Source: three-view drawing plus pictorial views. Frame: mm from the lowest corner of the part. A direction names the side the tool comes from. Round coordinates to 2 decimals unless told otherwise and drop trailing zeros. Loops run counter-clockwise (first coordinate to the right, second up) from the corner with the lowest first, then second, coordinate; pieces in that order, holes last. Notation, with made-up numbers: M 76,53 L 87,53 A17 cw 87,66 Z; hole C 60,-25 d11. An arc over 180 degrees is marked long. Write each question's results on one line, items separated by ' | '.
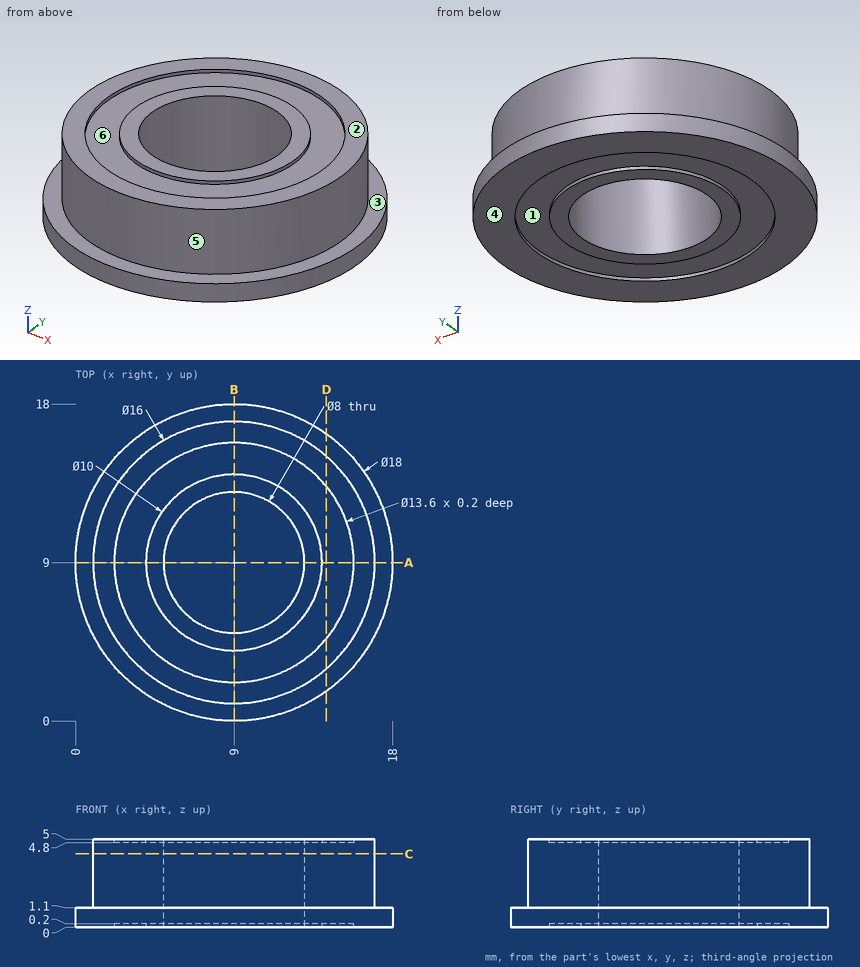
1. Access query for the marked faces 1, 2 and 3. Directions: +Z, -Z, +X, -X, +Y, -Y. A direction counts if a zero-diameter tool reaches every point of the face in a straight line with its end or side. Return the directions, or none.
Answer key:
face 1: -Z | face 2: +Z, +X, -X, +Y, -Y | face 3: +Z
2. Section D-D (x = 14.25). Output: boundary loops of the cut face in (y, z), then the cut area to 3 significant figures.
Answer key:
outline: M 1.69,0 L 4.68,0 L 4.68,0.2 L 13.32,0.2 L 13.32,0 L 16.31,0 L 16.31,1.1 L 15.04,1.1 L 15.04,5 L 13.32,5 L 13.32,4.8 L 4.68,4.8 L 4.68,5 L 2.96,5 L 2.96,1.1 L 1.69,1.1 Z | area: 59.7 mm²
3. Section C-C (z = 4.15). Output: boundary loops of the cut face in (x, y), then the cut area to 3 significant figures.
Answer key:
outline: C 9,9 d16; hole C 9,9 d8 | area: 151 mm²
4. Ray query, probe 1 along Y at (x, z) = (9, 0.15); probe 2 along Y at (x, z) = (9, 2.8); probe 3 along Y at (x, z) = (11.25, 2.2). Return the intervals inside material, ascending.
Answer key:
probe 1: y = 0 to 2.2, 4 to 5, 13 to 14, 15.8 to 18 | probe 2: y = 1 to 5, 13 to 17 | probe 3: y = 1.32 to 5.69, 12.31 to 16.68
5. Section A-A (y = 9). Output: boundary loops of the cut face in (x, z).
Answer key:
outline: M 0,0 L 2.2,0 L 2.2,0.2 L 4,0.2 L 4,0 L 5,0 L 5,5 L 4,5 L 4,4.8 L 2.2,4.8 L 2.2,5 L 1,5 L 1,1.1 L 0,1.1 Z; M 13,0 L 14,0 L 14,0.2 L 15.8,0.2 L 15.8,0 L 18,0 L 18,1.1 L 17,1.1 L 17,5 L 15.8,5 L 15.8,4.8 L 14,4.8 L 14,5 L 13,5 Z
6. Pin query (flat end, axial travel): P1, Ø9, axis at x = 5.5, y = 9, coming from the +Z side; P2, Ø6.5, axis at x = 9, y = 9, coming from the -Z side; P3, Ø1, axis at y = 2, z = 4.5, coming from the -X side. Return the tip coordinate at first contact, or that it passes through.
Answer key:
P1: stops at z = 5 | P2: passes through | P3: stops at x = 4.34
7. Draft query along Y for the marked faces 4, 5 and 6. Return one class per face: pulls with the +Y half, pulls with the -Y half, needs draft (parallel to the pull), parting line crosses it, or undercut.
Answer key:
face 4: needs draft | face 5: parting line crosses it | face 6: undercut
